Work out the finished part from the listing and answer in its coordinate system (mm). A direction names the side the tool comes from. Coordinates: 2 decimals unless noted, no trailing zeros. Order: outer loops, then holes, each group sorted by start corner. A loop starts at its lowest first (then second) coordinate and runs counter-clockwise, first axis right, second up.
```python
from build123d import *

# Parameters (mm, degrees)
BOSS_EXTRUDE1_DEPTH = 8
SKETCH2_R           = 2
CUT_EXTRUDE1_DEPTH  = 8
SKETCH3_W           = 8
SKETCH3_H           = 3
CUT_EXTRUDE2_DEPTH  = 2


with BuildPart() as part:
    # Sketch1 → Boss-Extrude1 (new body)
    with BuildSketch(Plane.XY):
        with BuildLine():
            Line((0.688022284, 7.008356546), (0.688022284, -15.991643454))
            ThreePointArc((0.688022284, -15.991643454), (9.688022284, -24.991643454), (0.688022284, -33.991643454))
            Line((0.688022284, -33.991643454), (0.688022284, -35.991643454))
            Line((0.688022284, -35.991643454), (17.688022284, -35.991643454))
            Line((17.688022284, -35.991643454), (17.688022284, 14.008356546))
            Line((17.688022284, 14.008356546), (0.688022284, 14.008356546))
            Line((0.688022284, 14.008356546), (0.688022284, 13.008356546))
            Line((0.688022284, 13.008356546), (4.46794824, 13.008356546))
            ThreePointArc((4.46794824, 13.008356546), (6.96794824, 10.508356546), (4.46794824, 8.008356546))
            Line((4.46794824, 8.008356546), (0.688022284, 8.008356546))
            Line((0.688022284, 8.008356546), (0.688022284, 7.008356546))
        make_face()
    extrude(amount=BOSS_EXTRUDE1_DEPTH)

    # Sketch2 → Cut-Extrude1 (cut)
    with BuildSketch(Plane.XY.offset(8)):
        with Locations((10.688022284, 10.508356546)):
            Circle(SKETCH2_R)
    extrude(amount=-CUT_EXTRUDE1_DEPTH, mode=Mode.SUBTRACT)

    # Sketch3 → Cut-Extrude2 (cut)
    with BuildSketch(Plane(origin=(0, 14.008356546, 0), x_dir=(1, 0, 0), z_dir=(0, 1, 0))):
        with Locations((4.688022284, -4)):
            Rectangle(SKETCH3_W, SKETCH3_H)
    extrude(amount=-CUT_EXTRUDE2_DEPTH, mode=Mode.SUBTRACT)


solid = part.part
```
1. The part is cut by section D-D (y = -27). Determine the outline of the cut face in (x, z), plus the area to 3 significant figures.
2. Consider probe 1 along Y at (x, z) = (10.5, 7.5); probe 2 along Y at (x, z) = (5.5, 2.25); probe 3 along Y at (x, z) = (11.25, 6.75). Determine where each line is inside the solid, lowest interval first.
3. The part is cut by section B-B (x = 3.75). Determine the outline of the cut face in (y, z).
4. The mould has two halves that part along X. Classify faces 4 (the cylindrical face through (9.1, 9.29, 4.06)), 5 (the flat face through (8.688, 13, 4)), 6 (the flat face through (3, 13.008, 7)): released by +X, released by -X, zero draft, split by the parting line, or undercut.
5. For faces 1 (the flat face through (3, 8.008, 4)), 2 (the flat face through (0.688, 13.5, 6.7)), 3 (the flat face through (6, 13, 5.5)), determine the directions among +Z, -Z, +X, -X, +Y, -Y from which every point of the face is accessible in a straight line to the end or side of a thin tool.
6. Flat-ended cylindrical pins translate along their axes: pin 1 (1.6 mm diameter, centred on y = 13, z = 3.5, fed in from -X); pin 2 (3.5 mm diameter, centred on x = 10.69, y = 10.51, fed in from -Z); pin 3 (0.7 mm diameter, centred on x = 7.5, z = 4.5, fed in from +Y); pin 4 (4 mm diameter, centred on x = 3.5, z = 3, fed in from +Y). Find the tip coordinate at first contact, or state that the pin passes through.
7. The part is cut by section C-C (z = 0.75). Determine the outline of the cut face in (x, y).
8. The part is cut by section A-A (x = 11). Determine the outline of the cut face in (y, z).
Worked out:
1. outline: (9.46, 0) - (17.69, 0) - (17.69, 8) - (9.46, 8) - close
1. area: 65.8 mm2
2. probe 1: y = -35.99 to 8.52, 12.5 to 14.01
2. probe 2: y = -35.99 to -32.6, -17.39 to 8.23, 12.79 to 14.01
2. probe 3: y = -35.99 to 8.59, 12.43 to 14.01
3. outline: (-35.99, 0) - (-33.45, 0) - (-33.45, 8) - (-35.99, 8) - close; (-16.53, 0) - (8.01, 0) - (8.01, 8) - (-16.53, 8) - close; (13.01, 0) - (14.01, 0) - (14.01, 2.5) - (13.01, 2.5) - close; (13.01, 5.5) - (14.01, 5.5) - (14.01, 8) - (13.01, 8) - close
4. face 4: undercut
4. face 5: released by -X
4. face 6: zero draft
5. face 1: +Z, -Z, -X
5. face 2: +Z, -Z, -X, +Y, -Y
5. face 3: -X, +Y
6. pin 1: stops at x = 8.69
6. pin 2: passes through
6. pin 3: stops at y = 12.01
6. pin 4: stops at y = 14.01
7. outline: (0.69, -35.99) - (17.69, -35.99) - (17.69, 14.01) - (0.69, 14.01) - (0.69, 13.01) - (4.47, 13.01) arc R2.5 cw to (4.47, 8.01) - (0.69, 8.01) - (0.69, -15.99) arc R9 cw to (0.69, -33.99) - close; hole circle Ø4 at (10.69, 10.51)
8. outline: (-35.99, 0) - (8.53, 0) - (8.53, 8) - (-35.99, 8) - close; (12.48, 0) - (14.01, 0) - (14.01, 8) - (12.48, 8) - close
